Source: CAD feature listing. Evaluate the final solid. Frame: model axes, mm. Face numbers are marked on the shaded views. A direction names the side the tool comes from. Round coordinates to 2 decimals unless told otherwise and drop trailing zeros. Loops run counter-clockwise (first coordinate to the right, second up) from the corner with the lowest first, then second, coordinate; pieces in that order, holes last. Notation, with made-up numbers: (46.5, 79) -> (93.5, 79) arc R17 ccw to (93.5, 83) -> close; hole circle Ø8 at (-1, -13). An arc over 180 degrees is marked (long way). Put each result on its own line as item: value. Start each with the question number.
1. Material intervals for L1, parallel to Z at x = 8.5, y = -15.1; L2, parallel to Y at x = 11, z = 38.5; L3, parallel to Z at x = 0, y = -13.1, sorted ascending.
2. Cut plane C-C (x = 8.5). Return the cut outline in (y, z).
3. Cut plane D-D (z = 19). State how many separate pieces and enclosed holes the cut face has, then the cut area to 3 significant figures.
4. Cut plane A-A (x = -11.5). Return the cut outline in (y, z), then the cut area to 3 significant figures.
5. Set-up query: the marked faces 1 and 2. Return all of +Z, -Z, +X, -X, +Y, -Y with unobstructed straight access to the full face (end or side cutting, diameter ignored); none if empty.
6. Contact query for flat-ended pins moving along their axis: pin 1 (3 mm diameter, centred on x = 12, y = 6.5, fed in from -Z); pin 2 (1.6 mm diameter, centred on y = 11.5, z = 21, fed in from -X); pin 3 (0.9 mm diameter, centred on x = -11.5, z = 23, fed in from +Y). Output: stop coordinate, or through.
7. Draft query along X for the marked faces 3 and 4. Return one class per face: pulls with the +X half, pulls with the -X half, needs draft (parallel to the pull), parting line crosses it, or undercut.
8. Cut plane B-B (y = 0). Return the cut outline in (x, z), then the cut area to 3 significant figures.
```python
from build123d import *

# Parameters (mm, degrees)
F0_W     = 1
F0_H     = 1.5
F0_W_2   = 2
F0_H_2   = 2
F0_W_3   = 4.75
F0_W_4   = 1.5
F0_H_3   = 1
F0_H_4   = 2.8
F0_R     = 6
F1_DEPTH = 50
F3_D     = 5.1054
F3_DEPTH = 8.89
F3_TIP   = 1.5338169022
F4_D     = 2.5
F4_DEPTH = 4.675
F4_TIP   = 0.7510757738


with BuildPart() as f1:
    # F0 (on Top) → F1 (new body)
    with BuildSketch(Plane.XY):
        with Locations((-10, 15.75)):
            Rectangle(F0_W, F0_H)
        with Locations((-7.25, 15.75)):
            Rectangle(F0_W, F0_H)
        with Locations((-4.5, 15.75)):
            Rectangle(F0_W, F0_H)
        with Locations((4.5, 15.75)):
            Rectangle(F0_W, F0_H)
        with Locations((7.25, 15.75)):
            Rectangle(F0_W, F0_H)
        with Locations((10, 15.75)):
            Rectangle(F0_W, F0_H)
        Polygon((16.5, 13), (16.5, 16.5), (13, 16.5), (13, 15), (15, 15), (15, 13), align=None)
        with Locations((14, 14)):
            Rectangle(F0_W_2, F0_H_2)
        Polygon((13, 13), (13, 15), (10.5, 15), (9.5, 15), (7.75, 15), (6.75, 15), (5, 15), (4, 15), (2.375, 15), (2.375, 13), align=None)
        with Locations((0, 14)):
            Rectangle(F0_W_3, F0_H_2)
        with Locations((0, 15.75)):
            Rectangle(F0_W_3, F0_H)
        Polygon((-13, 13), (-2.375, 13), (-2.375, 15), (-4, 15), (-5, 15), (-6.75, 15), (-7.75, 15), (-9.5, 15), (-10.5, 15), (-13, 15), align=None)
        with Locations((-14, 14)):
            Rectangle(F0_W_2, F0_H_2)
        Polygon((-16.5, 13), (-15, 13), (-15, 15), (-13, 15), (-13, 16.5), (-16.5, 16.5), align=None)
        Polygon((-13, 1.4), (-13, 13), (-15, 13), (-15, 10.5), (-15, 9.5), (-15, 7.75), (-15, 6.75), (-15, 5), (-15, 4), (-15, 1.4), align=None)
        with Locations((-15.75, 10)):
            Rectangle(F0_W_4, F0_H_3)
        with Locations((-15.75, 7.25)):
            Rectangle(F0_W_4, F0_H_3)
        with Locations((-15.75, 4.5)):
            Rectangle(F0_W_4, F0_H_3)
        with Locations((-15.75, 0)):
            Rectangle(F0_W_4, F0_H_4)
        with Locations((-15.75, -4.5)):
            Rectangle(F0_W_4, F0_H_3)
        with Locations((-15.75, -7.25)):
            Rectangle(F0_W_4, F0_H_3)
        with Locations((-15.75, -10)):
            Rectangle(F0_W_4, F0_H_3)
        Polygon((-2.375, -15), (-2.375, -13), (-13, -13), (-13, -1.4), (-15, -1.4), (-15, -4), (-15, -5), (-15, -6.75), (-15, -7.75), (-15, -9.5), (-15, -10.5), (-15, -15), align=None)
        with Locations((-14, 0)):
            Rectangle(F0_W_2, F0_H_4)
        with BuildLine():
            ThreePointArc((-9.9015150356, -1.4), (-10, 0), (-9.9015150356, 1.4))
            Line((-9.9015150356, 1.4), (-13, 1.4))
            Line((-13, 1.4), (-13, -1.4))
            Line((-13, -1.4), (-9.9015150356, -1.4))
        make_face()
        with BuildLine():
            Line((2.375, 9.7138753852), (2.375, 13))
            Line((2.375, 13), (-2.375, 13))
            Line((-2.375, 13), (-2.375, 9.7138753852))
            ThreePointArc((-2.375, 9.7138753852), (0, 10), (2.375, 9.7138753852))
        make_face()
        with BuildLine():
            Line((13, -1.4), (13, 1.4))
            Line((13, 1.4), (9.9015150356, 1.4))
            ThreePointArc((9.9015150356, 1.4), (9.9753483738, 0.7017298783), (10, 0))
            ThreePointArc((10, 0), (9.9753483738, -0.7017298783), (9.9015150356, -1.4))
            Line((9.9015150356, -1.4), (13, -1.4))
        make_face()
        with Locations((14, 0)):
            Rectangle(F0_W_2, F0_H_4)
        with Locations((15.75, 10)):
            Rectangle(F0_W_4, F0_H_3)
        with Locations((15.75, 7.25)):
            Rectangle(F0_W_4, F0_H_3)
        with Locations((15.75, 4.5)):
            Rectangle(F0_W_4, F0_H_3)
        with Locations((15.75, 0)):
            Rectangle(F0_W_4, F0_H_4)
        Polygon((15, 10.5), (15, 13), (13, 13), (13, 1.4), (15, 1.4), (15, 4), (15, 5), (15, 6.75), (15, 7.75), (15, 9.5), align=None)
        Polygon((15, -1.4), (13, -1.4), (13, -13), (2.375, -13), (2.375, -15), (15, -15), (15, -10.5), (15, -9.5), (15, -7.75), (15, -6.75), (15, -5), (15, -4), align=None)
        with Locations((15.75, -4.5)):
            Rectangle(F0_W_4, F0_H_3)
        with Locations((15.75, -7.25)):
            Rectangle(F0_W_4, F0_H_3)
        with Locations((15.75, -10)):
            Rectangle(F0_W_4, F0_H_3)
        with Locations((0, -14)):
            Rectangle(F0_W_3, F0_H_2)
        with Locations((0, -15.75)):
            Rectangle(F0_W_3, F0_H)
        Polygon((15, -15), (2.375, -15), (2.375, -16.5), (16.5, -16.5), (16.5, -15), align=None)
        Polygon((-2.375, -16.5), (-2.375, -15), (-15, -15), (-16.5, -15), (-16.5, -16.5), align=None)
        with BuildLine():
            Line((2.375, -13), (2.375, -9.7138753852))
            ThreePointArc((2.375, -9.7138753852), (0, -10), (-2.375, -9.7138753852))
            Line((-2.375, -9.7138753852), (-2.375, -13))
            Line((-2.375, -13), (2.375, -13))
        make_face()
        with BuildLine():
            ThreePointArc((10, 0), (9.9753483738, 0.7017298783), (9.9015150356, 1.4))
            ThreePointArc((9.9015150356, 1.4), (7.4133889912, 6.7113086403), (2.375, 9.7138753852))
            ThreePointArc((2.375, 9.7138753852), (0, 10), (-2.375, 9.7138753852))
            ThreePointArc((-2.375, 9.7138753852), (-7.4133889912, 6.7113086403), (-9.9015150356, 1.4))
            ThreePointArc((-9.9015150356, 1.4), (-10, 0), (-9.9015150356, -1.4))
            ThreePointArc((-9.9015150356, -1.4), (-7.4133889912, -6.7113086403), (-2.375, -9.7138753852))
            ThreePointArc((-2.375, -9.7138753852), (0, -10), (2.375, -9.7138753852))
            ThreePointArc((2.375, -9.7138753852), (7.4133889912, -6.7113086403), (9.9015150356, -1.4))
            ThreePointArc((9.9015150356, -1.4), (9.9753483738, -0.7017298783), (10, 0))
        make_face()
        Circle(F0_R, mode=Mode.SUBTRACT)
    extrude(amount=F1_DEPTH)

    # F3
    with Locations(Plane.XZ.offset(16.5)):
        with Locations((0, 25)):
            Hole(F3_D / 2, depth=F3_DEPTH)
            with Locations((0, 0, -(F3_DEPTH + F3_TIP / 2))):  # 118° drill point
                Cone(0, F3_D / 2, F3_TIP, mode=Mode.SUBTRACT)

    # F4
    with Locations(Plane.XZ.offset(16.5)):
        with Locations((-8.5, 45), (0, 45), (0, 41), (8.5, 45), (8.5, 5), (0, 5), (-8.5, 5)):
            Hole(F4_D / 2, depth=F4_DEPTH)
            with Locations((0, 0, -(F4_DEPTH + F4_TIP / 2))):  # 118° drill point
                Cone(0, F4_D / 2, F4_TIP, mode=Mode.SUBTRACT)


solid = f1.part
```
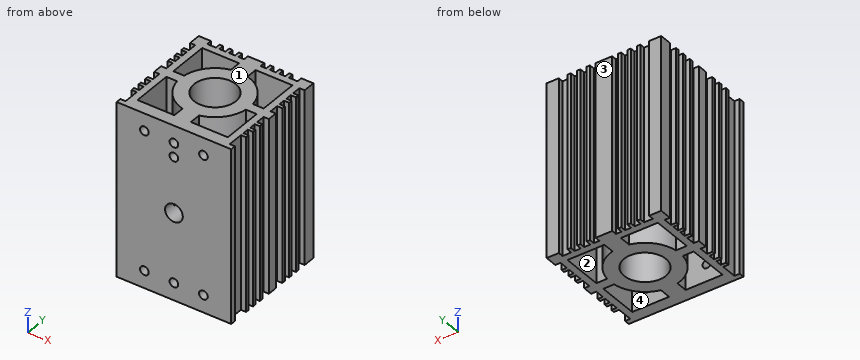
Solution:
1. L1: z = 0 to 3.75, 6.25 to 43.75, 46.25 to 50
1. L2: y = -16.5 to -13, -1.4 to 1.4, 13 to 15
1. L3: z = 0 to 3.75, 6.25 to 22.45, 27.55 to 39.75, 42.25 to 43.75, 46.25 to 50
2. outline: (-16.5, 0) -> (-13, 0) -> (-13, 3.75) -> (-16.5, 3.75) -> close; (-16.5, 6.25) -> (-13, 6.25) -> (-13, 43.75) -> (-16.5, 43.75) -> close; (-16.5, 46.25) -> (-13, 46.25) -> (-13, 50) -> (-16.5, 50) -> close; (-5.27, 0) -> (5.27, 0) -> (5.27, 50) -> (-5.27, 50) -> close; (13, 0) -> (15, 0) -> (15, 50) -> (13, 50) -> close
3. separate pieces: 1
3. enclosed holes: 5
3. area: 580 mm^2
4. outline: (-16.5, 0) -> (-13, 0) -> (-13, 50) -> (-16.5, 50) -> close; (-1.4, 0) -> (1.4, 0) -> (1.4, 50) -> (-1.4, 50) -> close; (13, 0) -> (15, 0) -> (15, 50) -> (13, 50) -> close
4. area: 415 mm^2
5. face 1: +Z, +X, -X, +Y, -Y
5. face 2: +Z, -Z
6. pin 1: stops at z = 0
6. pin 2: stops at x = -15
6. pin 3: stops at y = 15
7. face 3: needs draft
7. face 4: undercut
8. outline: (-16.5, 0) -> (-6, 0) -> (-6, 50) -> (-16.5, 50) -> close; (6, 0) -> (16.5, 0) -> (16.5, 50) -> (6, 50) -> close
8. area: 1,050 mm^2
